Build history of the part. All positions in model axes, mm. A direction names the side the tool comes from. Give positions to 0.01 mm unless a question says otherwise; leave off trailing zeros. Loops run counter-clockwise (first coordinate to the right, second up) from the corner with the lowest first, then second, coordinate; pieces in that order, holes last. Notation, with made-up numbers: (-40, 69) -> (-31, 69) arc R16 cw to (-31, 80) -> close; hole circle Ø11 at (23, -0.75). An arc over 180 degrees is marked (long way). Answer as a JSON object with one key per item and string values. Group by question number.
from build123d import *

# Parameters (mm, degrees)
F0_W     = 25
F0_H     = 3.75
F3_DEPTH = 50.001
F4_R     = 1
F2_R     = 10
F5_DEPTH = 1


with BuildPart() as f1:
    # F0 (on Front) → F1 (revolve)
    with BuildSketch(Plane.XZ):
        Polygon((-50, 0), (-38, 0), (-38, 10), (-38, 21.5), (-50, 21.5), align=None)
        Polygon((-38, 0), (-25, 0), (-25, 3.75), (-25, 10), (-38, 10), align=None)
        with Locations((-12.5, 1.875)):
            Rectangle(F0_W, F0_H)
    revolve(axis=Axis((-31.744454056, 0, 0), (-1, 0, 0)))

    # F2 (on face) → F3 (cut, through all)
    with BuildSketch(Plane(origin=(-50, 0, 0), x_dir=(0, -1, 0), z_dir=(-1, 0, 0))):
        with BuildLine():
            ThreePointArc((-21.4064859646, 2.0030872791), (-7.8523074483, 7.8523074483), (-2.0030872791, 21.4064859646))
            ThreePointArc((-2.0030872791, 21.4064859646), (-15.2027957955, 15.2027957955), (-21.4064859646, 2.0030872791))
        make_face()
        with BuildLine():
            ThreePointArc((2.0030872791, 21.4064859646), (7.8523074483, 7.8523074483), (21.4064859646, 2.0030872791))
            ThreePointArc((21.4064859646, 2.0030872791), (15.2027957955, 15.2027957955), (2.0030872791, 21.4064859646))
        make_face()
        with BuildLine():
            ThreePointArc((-21.4064859646, -2.0030872791), (-15.2027957955, -15.2027957955), (-2.0030872791, -21.4064859646))
            ThreePointArc((-2.0030872791, -21.4064859646), (-7.8523074483, -7.8523074483), (-21.4064859646, -2.0030872791))
        make_face()
        with BuildLine():
            ThreePointArc((2.0030872791, -21.4064859646), (15.2027957955, -15.2027957955), (21.4064859646, -2.0030872791))
            ThreePointArc((21.4064859646, -2.0030872791), (7.8523074483, -7.8523074483), (2.0030872791, -21.4064859646))
        make_face()
    extrude(amount=-F3_DEPTH, mode=Mode.SUBTRACT)

    # F4
    f4_edges = [f1.edges().sort_by_distance(p)[0] for p in [
        (-50, -7.852307, 7.852307),
        (-50, 0, 21.5),
        (-50, 7.852307, 7.852307),
        (-50, 21.5, 0),
        (-50, 7.852307, -7.852307),
        (-50, 0, -21.5),
        (-50, -7.852307, -7.852307),
        (-50, -21.5, 0),
        (-44, -2.003087, -21.406486),
        (-44, 21.406486, -2.003087),
        (-44, -21.406486, -2.003087),
        (-44, -2.003087, 21.406486),
        (-44, -21.406486, 2.003087),
        (-44, 2.003087, 21.406486),
        (-44, 21.406486, 2.003087),
        (-44, 2.003087, -21.406486),
        (-25, 0, -10),
    ]]
    fillet(f4_edges, radius=F4_R)

    # F2 (on face) → F5 (cut)
    with BuildSketch(Plane(origin=(-50, 0, 0), x_dir=(0, -1, 0), z_dir=(-1, 0, 0))):
        Circle(F2_R)
    extrude(amount=-F5_DEPTH, mode=Mode.SUBTRACT)


solid = f1.part
(1) 3-axis set-ups, long thin cutter, end or side, ignore diameter. For faces 1 (the flat face through (-25, -4, 0)), 2 (the cylindrical face through (-43.577, -7.994, -7.712)), 3 (the cylindrical face through (-49.51, 2.17, -9.76)): which of +Z, -Z, +X, -X, +Y, -Y reach the whole face in a straight line?
(2) Saw through at A-A on z = 0. List the corners of the cut face in (x, y), plus the area to 3 significant figures.
(3) Pin check, flat tips, straight feed: pin 1 (4 mm diameter, centred on y = 9.5, z = -12, fed in from -X); pin 2 (8 mm diameter, centred on x = -24, z = 4.5, fed in from +Y); pin 3 (3 mm diameter, centred on x = -39, z = -13, fed in from -Y); pin 4 (12 mm diameter, centred on x = -8, y = -2.5, fed in from -Z). Stop position of each tip, or through.
(4) Saw through at D-D on x = -27.5. List the corners of the cut face in (y, z).
(5) Saw through at C-C on x = -8.5. List the corners of the cut face in (y, z).
(6) Pull direction Y, two halves, no side cores. Call faces 4 (the cylindrical face through (-43.577, 7.712, -7.994)), 5 (the flat face through (-49, 0, 0)), 6 (the flat face through (0, 0, 0)): pulls with the +Y half, pulls with the -Y half, needs draft (parallel to the pull), parting line crosses it, or undercut.
(7) Probe line 1 along X through (y, z) = (-1, -6); line 2 along Z through (x, y) = (-29, 7); line 3 along X through (y, z) = (-17, 2). List the from-to ranges inside material, lowest first. Write a range as [from, to].
Calculated:
{
 "1": {"face 1": "+X", "face 2": "-Z, +X, -X, -Y", "face 3": "-X"},
 "2": {"outline": "(-50, -20.5) arc R1 ccw to (-49, -21.5) -> (-38, -21.5) -> (-38, -10) -> (-26, -10) arc R1 ccw to (-25, -9) -> (-25, -3.75) -> (0, -3.75) -> (0, 3.75) -> (-25, 3.75) -> (-25, 9) arc R1 ccw to (-26, 10) -> (-38, 10) -> (-38, 21.5) -> (-49, 21.5) arc R1 ccw to (-50, 20.5) -> (-50, 10) -> (-49, 10) -> (-49, -10) -> (-50, -10) -> close", "area": "943 mm^2"},
 "3": {"pin 1": "passes through", "pin 2": "stops at y = 9.95", "pin 3": "stops at y = -4.97", "pin 4": "stops at z = -3.75"},
 "4": {"outline": "circle Ø20 at (0, 0)"},
 "5": {"outline": "circle Ø7.5 at (0, 0)"},
 "6": {"face 4": "pulls with the +Y half", "face 5": "undercut", "face 6": "needs draft"},
 "7": {"line 1": "x = [-49, -25]", "line 2": "z = [-7.14, 7.14]", "line 3": "x = [-49.92, -38]"}
}
